For this review, take the finished solid that the model builds, in its own axes (mm). A direction names the side the tool comes from. Round coordinates to 2 decimals unless told otherwise and drop trailing zeros. Order: outer loops, then holes, each group sorted by start corner. A loop starts at its lowest first (then second) coordinate and runs counter-clockwise, first axis right, second up. Notation, with made-up numbers: M -6,-1 L 27,-1 A18 cw 27,3 Z; hole C 9.5,21 d7. An arc over 180 degrees is marked long. Answer as a JSON object with one key per item and string values.
from build123d import *

# Parameters (mm, degrees)
SKETCH_1_R      = 12.5
EXTRUDE_1_DEPTH = 2
SKETCH_2_R      = 13
SKETCH_2_R_2    = 12.5
EXTRUDE_2_DEPTH = 5
SKETCH_3_R      = 14
SKETCH_3_R_2    = 12.5
EXTRUDE_3_DEPTH = 5


with BuildPart() as part:
    # 草圖1 → 填料-伸長1 (new body)
    with BuildSketch(Plane(origin=(0, 0, 0), x_dir=(1, 0, 0), z_dir=(0, 1, 0))):
        Polygon((-4.468973219, -15.535817059), (11.219925632, -11.638152866), (15.688898852, 3.897664193), (4.468973219, 15.535817059), (-11.219925632, 11.638152866), (-15.688898852, -3.897664193), align=None)
        with Locations(Location((0, 0, 0), (0, 0, 270))):
            Circle(SKETCH_1_R, mode=Mode.SUBTRACT)
    extrude(amount=EXTRUDE_1_DEPTH)

    # 草圖2 → 填料-伸長2 (add)
    with BuildSketch(Plane(origin=(0, 2, 0), x_dir=(1, 0, 0), z_dir=(0, 1, 0))):
        with Locations(Location((0, 0, 0), (0, 0, 270))):
            Circle(SKETCH_2_R)
        with Locations(Location((0, 0, 0), (0, 0, 270))):
            Circle(SKETCH_2_R_2, mode=Mode.SUBTRACT)
    extrude(amount=EXTRUDE_2_DEPTH)

    # 草圖3 → 填料-伸長3 (add)
    with BuildSketch(Plane(origin=(0, 7, 0), x_dir=(1, 0, 0), z_dir=(0, 1, 0))):
        with Locations(Location((0, 0, 0), (0, 0, 270))):
            Circle(SKETCH_3_R)
        with Locations(Location((0, 0, 0), (0, 0, 270))):
            Circle(SKETCH_3_R_2, mode=Mode.SUBTRACT)
    extrude(amount=EXTRUDE_3_DEPTH)


solid = part.part
1) Add section D-D on y = 5.5. State the section outline as (x, z) points.
Geometry check:
{"outline": "C 0,0 d26; hole C 0,0 d25"}
2) Add section A-A on x = -10.5. State the section outline as (y, z) points.
Geometry check:
{"outline": "M 0,-11.82 L 2,-11.82 L 2,-7.66 L 7,-7.66 L 7,-9.26 L 12,-9.26 L 12,-6.78 L 0,-6.78 Z; M 0,6.78 L 12,6.78 L 12,9.26 L 7,9.26 L 7,7.66 L 2,7.66 L 2,9.28 L 0,9.28 Z"}
3) Machinability: for faces 4 (the cylindrical face through (-7.91, 4.465, -10.316)), 5 (the cylindrical face through (3.755, 5.916, 11.923)), 6 (the cylindrical face through (-13.67, 9.46, -3.03)), which of the approach directions +Z, -Z, +X, -X, +Y, -Y give a long, thin tool a straight path to every point of the face, cutting with its end or side? Answer none if there is none.
Geometry check:
{"face 4": "none", "face 5": "+Y, -Y", "face 6": "+Y"}
4) For L1, parallel to X at y = 6.75, z = 0; L2, parallel to Y at x = 12.5, z = 7; L3, parallel to Z at x = 1, y = 4.25, list the stretches that pass through material, from the lowest coordinate up.
Geometry check:
{"L1": "x = -13 to -12.5, 12.5 to 13", "L2": "y = 0 to 2", "L3": "z = -12.96 to -12.46, 12.46 to 12.96"}
5) Add section C-C on y = 10.5. State the section outline as (x, z) points.
Geometry check:
{"outline": "C 0,0 d28; hole C 0,0 d25"}
6) Add section B-B on z = 0. State the section outline as (x, y) points.
Geometry check:
{"outline": "M -14.57,0 L -12.5,0 L -12.5,12 L -14,12 L -14,7 L -13,7 L -13,2 L -14.57,2 Z; M 12.5,0 L 14.57,0 L 14.57,2 L 13,2 L 13,7 L 14,7 L 14,12 L 12.5,12 Z"}
7) Mouldability with a two-part tool opening along Y and no side actions: class faces 1 (the flat face through (11.5, 12, -5.3)), 2 (the flat face through (-13.423, 0.986, -3.979)), 3 (the flat face through (-12, 2, 6)) as +Y half, -Y half, draft (parallel to the pull), parting line (faces both ways), or undercut.
Geometry check:
{"face 1": "+Y half", "face 2": "draft", "face 3": "undercut"}
8) Insertion check: P1, Ø10, axis at x = -7, z = -2.5, coming from the -Y side; P2, Ø1.5, axis at y = 7.5, z = 10.5, coming from the -X side; P3, Ø6, axis at x = -9.5, z = -3.5, coming from the -Y side; P4, Ø1.5, axis at x = 8.5, y = 5, coming from the -Z side. Each pin has a flat end and moves straight along its axis. Give the tip position at first contact, or say it passes through.
Geometry check:
{"P1": "passes through", "P2": "stops at x = -10.05", "P3": "stops at y = 0", "P4": "stops at z = -10.44"}
